```python
from build123d import *

# Parameters (mm, degrees)
SKETCH1_W           = 57.5
SKETCH1_H           = 109
SKETCH1_R           = 1.75
SKETCH1_W_2         = 28.5
SKETCH1_H_2         = 95
BOSS_EXTRUDE1_DEPTH = 1.5
SKETCH3_W           = 43.5
SKETCH3_H           = 81
CUT_EXTRUDE1_DEPTH  = 3
BOSS_EXTRUDE2_DEPTH = 85
SKETCH5_W           = 145.39083122
SKETCH5_H           = 125.853938275
CUT_EXTRUDE2_DEPTH  = 85
CUT_EXTRUDE3_DEPTH  = 140.802762848
SKETCH8_W           = 103
SKETCH8_H           = 3
BOSS_EXTRUDE3_DEPTH = 25.75
FILLET3_R           = 3
SKETCH13_W          = 109
SKETCH13_H          = 88
CUT_EXTRUDE8_DEPTH  = 1.75
SKETCH14_W          = 2
SKETCH14_H          = 25
CUT_EXTRUDE9_DEPTH  = 5
SKETCH15_W          = 7
SKETCH15_H          = 25
CUT_EXTRUDE10_DEPTH = 106.016665344
SKETCH16_W          = 3
SKETCH16_H          = 15
BOSS_EXTRUDE4_DEPTH = 5
SKETCH17_W          = 7.5
SKETCH17_H          = 4
BOSS_EXTRUDE5_DEPTH = 3
CHAMFER1_SIZE       = 2
SKETCH18_R          = 10
CUT_EXTRUDE11_DEPTH = 10


with BuildPart() as part:
    # Sketch1 → Boss-Extrude1 (new, symmetric)
    with BuildSketch(Plane(origin=(0, 0, 0), x_dir=(1, 0, 0), z_dir=(0, 1, 0))):
        Rectangle(SKETCH1_W, SKETCH1_H)
        with Locations(Location((-21.25, 47, 0), (0, 0, 270))):
            Circle(SKETCH1_R, mode=Mode.SUBTRACT)
        with Locations(Location((21.25, 47, 0), (0, 0, 270))):
            Circle(SKETCH1_R, mode=Mode.SUBTRACT)
        with Locations(Location((21.25, -47, 0), (0, 0, 270))):
            Circle(SKETCH1_R, mode=Mode.SUBTRACT)
        with Locations(Location((-21.25, -47, 0), (0, 0, 270))):
            Circle(SKETCH1_R, mode=Mode.SUBTRACT)
        Rectangle(SKETCH1_W_2, SKETCH1_H_2, mode=Mode.SUBTRACT)
    extrude(amount=BOSS_EXTRUDE1_DEPTH, both=True)

    # Sketch3 → Cut-Extrude1 (cut)
    with BuildSketch(Plane(origin=(0, 1.5, 0), x_dir=(1, 0, 0), z_dir=(0, 1, 0))):
        Rectangle(SKETCH3_W, SKETCH3_H)
    extrude(amount=-CUT_EXTRUDE1_DEPTH, mode=Mode.SUBTRACT)

    # Sketch4 → Boss-Extrude2 (add)
    with BuildSketch(Plane.XZ.offset(1.5)):
        Polygon((28.75, 54.5), (27.30464021, 54.5), (-28.75, 54.5), (-28.75, 51.5), (25.75, 51.5), (25.75, -51.5), (-28.75, -51.5), (-28.75, -54.5), (27.30464021, -54.5), (28.75, -54.5), align=None)
    extrude(amount=BOSS_EXTRUDE2_DEPTH)

    # Sketch5 → Cut-Extrude2 (cut)
    with BuildSketch(Plane(origin=(0, 0, 0), x_dir=(0, 0, -1), z_dir=(1, 0, 0))):
        with Locations((7.269541561, -54.313017537)):
            Rectangle(SKETCH5_W, SKETCH5_H)
    extrude(amount=-CUT_EXTRUDE2_DEPTH, mode=Mode.SUBTRACT)

    # Sketch6 → Cut-Extrude3 (cut, through all)
    with BuildSketch(Plane(origin=(0, 0, 51.5), x_dir=(-1, 0, 0), z_dir=(0, 0, -1))):
        Polygon((0, -6.5), (-20.75, -27.25), (-20.75, -57.75), (0, -78.5), align=None)
    extrude(amount=CUT_EXTRUDE3_DEPTH, mode=Mode.SUBTRACT)

    # Sketch8 → Boss-Extrude3 (add)
    with BuildSketch(Plane.ZY.offset(-25.75)):
        with Locations((0, -85)):
            Rectangle(SKETCH8_W, SKETCH8_H)
    extrude(amount=BOSS_EXTRUDE3_DEPTH)

    # Fillet3
    fillet3_edges = [part.edges().sort_by_distance(p)[0] for p in [
        (0, 0, -47.5),
        (0, 0, 47.5),
        (0, -78.5, -53),
        (20.75, -27.25, -53),
        (0, -6.5, -53),
        (20.75, -57.75, -53),
        (14.25, 0, 47.5),
        (14.25, 0, -47.5),
        (21.75, 0, 40.5),
        (21.75, 0, -40.5),
    ]]
    fillet(fillet3_edges, radius=FILLET3_R)

    # Sketch13 → Cut-Extrude8 (cut)
    with BuildSketch(Plane.ZY):
        with Locations((0, -42.5)):
            Rectangle(SKETCH13_W, SKETCH13_H)
    extrude(amount=-CUT_EXTRUDE8_DEPTH, mode=Mode.SUBTRACT)

    # Sketch14 → Cut-Extrude9 (cut)
    with BuildSketch(Plane.XY.offset(54.5)):
        with Locations((2.75, -28)):
            Rectangle(SKETCH14_W, SKETCH14_H)
    extrude(amount=-CUT_EXTRUDE9_DEPTH, mode=Mode.SUBTRACT)

    # Sketch15 → Cut-Extrude10 (cut, through all)
    with BuildSketch(Plane.ZY.offset(-25.75)):
        with Locations((47, -14)):
            Rectangle(SKETCH15_W, SKETCH15_H)
        with Locations((-47, -14)):
            Rectangle(SKETCH15_W, SKETCH15_H)
    extrude(amount=-CUT_EXTRUDE10_DEPTH, mode=Mode.SUBTRACT)

    # Sketch16 → Boss-Extrude4 (add)
    with BuildSketch(Plane(origin=(0, 1.5, 0), x_dir=(1, 0, 0), z_dir=(0, 1, 0))):
        with Locations((12.75, 44)):
            Rectangle(SKETCH16_W, SKETCH16_H)
        with Locations((12.75, -44)):
            Rectangle(SKETCH16_W, SKETCH16_H)
    extrude(amount=-BOSS_EXTRUDE4_DEPTH)

    # Sketch17 → Boss-Extrude5 (add)
    with BuildSketch(Plane(origin=(0, 1.5, 0), x_dir=(1, 0, 0), z_dir=(0, 1, 0))):
        with Locations((18, 38.5)):
            Rectangle(SKETCH17_W, SKETCH17_H)
        with Locations((18, -38.5)):
            Rectangle(SKETCH17_W, SKETCH17_H)
    extrude(amount=-BOSS_EXTRUDE5_DEPTH)

    # Chamfer1
    chamfer1_edges = [part.edges().sort_by_distance(p)[0] for p in [
        (14.25, -1.5, 44),
        (14.25, -1.5, -44),
    ]]
    chamfer(chamfer1_edges, length=CHAMFER1_SIZE - 0.0001)  # a hair under: the kernel refuses the full size

    # Sketch18 → Cut-Extrude11 (cut)
    with BuildSketch(Plane.XZ.offset(86.5)):
        with Locations((1.75, 34.5)):
            Circle(SKETCH18_R)
    extrude(amount=-CUT_EXTRUDE11_DEPTH, mode=Mode.SUBTRACT)


solid = part.part
```
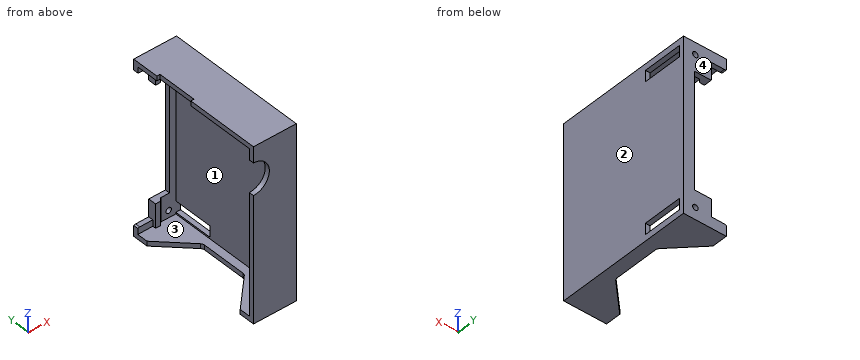
The model under review builds one solid part; all positions refer to its coordinate system, in mm. Face numbers are marked on the shaded views. Round coordinates to 2 decimals unless told otherwise and drop trailing zeros. Loops run counter-clockwise (first coordinate to the right, second up) from the corner with the lowest first, then second, coordinate; pieces in that order, holes last.
1) Clearance check with flat-ended pins moving along their axes: P1, Ø1.5, axis at y = -18, z = -23.5, coming from the -X side; P2, Ø2.5, axis at y = -1, z = 45, coming from the -X side; P3, Ø1.5, axis at y = -40, z = -52.5, coming from the -X side. State where each tip first meets the part, or that it passes through.
Values follow:
P1: stops at x = 25.75
P2: stops at x = 11.25
P3: stops at x = 20.75
2) Consider section A-A on x = 17.5. State the section outline as (y, z) points, then the cut area to 3 significant figures.
Values follow:
outline: (-86.5, -54.5) - (-61, -54.5) - (-61, -51.5) - (-83.5, -51.5) - (-83.5, 51.5) - (-1.5, 51.5) - (-1.5, 36.5) - (1.5, 36.5) - (1.5, 54.5) - (-86.5, 54.5) - close; (-24, -54.5) - (1.5, -54.5) - (1.5, -36.5) - (-1.5, -36.5) - (-1.5, -51.5) - (-24, -51.5) - close
area: 816 mm2
3) Wall thickness on line 1 along Z through (x, y) = (12.75, -13); line 2 along X through (y, z) = (-0.05, -47); line 3 along Y through (x, z) = (25.25, -44): over which ranges is each line inside the solid? List them lowest first.
Values follow:
line 1: z = -54.5 to -51.5, 51.5 to 54.5
line 2: x = 11.25 to 19.5, 23 to 28.75
line 3: y = -86.5 to -83.5, -1.5 to 1.5
4) The part is to be moulded in two halves that separate along Y. For the marked faces 1, 2, 3 and 4, say which applies: pulls with the +Y half, pulls with the -Y half, needs draft (parallel to the pull), parting line crosses it, or undercut.
Values follow:
face 1: undercut
face 2: needs draft
face 3: undercut
face 4: pulls with the +Y half
5) Consider section C-C on y = -80.5. State the section outline as (x, z) points.
Values follow:
outline: (1.75, -54.5) - (28.75, -54.5) - (28.75, 54.5) - (1.75, 54.5) - (1.75, 51.5) - (25.75, 51.5) - (25.75, -51.5) - (1.75, -51.5) - close
6) Consider section B-B on z = 34.5. State the section outline as (x, y) points.
Values follow:
outline: (11.75, -86.5) - (28.75, -86.5) - (28.75, 1.5) - (21.75, 1.5) - (21.75, -1.5) - (25.75, -1.5) - (25.75, -83.5) - (11.75, -83.5) - close
